CAD build for the part. Positions are in the model's coordinates, mm. Face numbers are marked on the shaded views. A direction names the side the tool comes from. Coordinates: 2 decimals unless noted, no trailing zeros. Order: outer loops, then holes, each group sorted by start corner. A loop starts at its lowest first (then second) coordinate and runs counter-clockwise, first axis right, second up. Notation, with made-up numbers: M 49,80.25 L 70,80.25 A24 cw 70,97.25 Z; hole C 36.25,-25.5 d3. An arc over 180 degrees is marked long. Write item = value, one per line.
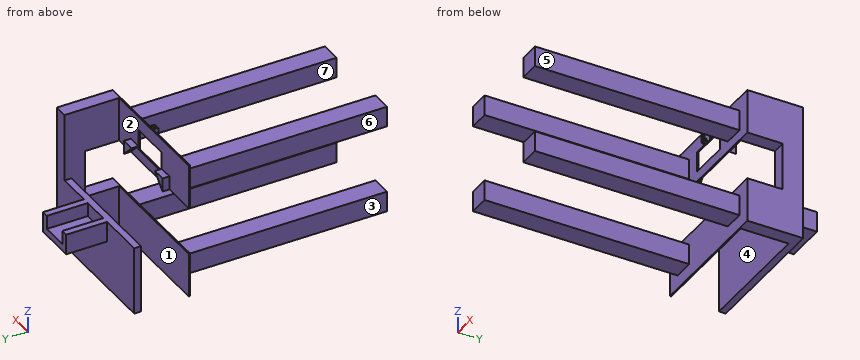
from build123d import *

# Parameters (mm, degrees)
SKETCH1_W           = 1000
SKETCH1_H           = 1000
BOSS_EXTRUDE1_DEPTH = 10
SKETCH5_W           = 150
SKETCH5_H           = 150
BOSS_EXTRUDE2_DEPTH = 1500
SKETCH7_W           = 300
SKETCH7_H           = 150
CUT_EXTRUDE1_DEPTH  = 1500
SKETCH9_W           = 10
SKETCH9_H           = 120
BOSS_EXTRUDE4_DEPTH = 40
FILLET1_R           = 10
FILLET2_R           = 10
SKETCH10_R          = 5
CUT_EXTRUDE3_DEPTH  = 55
SKETCH11_W          = 100
SKETCH11_H          = 1000
BOSS_EXTRUDE5_DEPTH = 400
SKETCH12_W          = 500
SKETCH12_H          = 50
BOSS_EXTRUDE6_DEPTH = 900
SKETCH14_W          = 300
SKETCH14_H          = 150
BOSS_EXTRUDE7_DEPTH = 300
SKETCH15_W          = 200
SKETCH15_H          = 100
CUT_EXTRUDE4_DEPTH  = 300
SKETCH8_W           = 1000
SKETCH8_H           = 350
CUT_EXTRUDE2_DEPTH  = 2069.840254829
SKETCH16_W          = 350
SKETCH16_H          = 250
CUT_EXTRUDE5_DEPTH  = 2062.552812809
BOSS_EXTRUDE8_DEPTH = 50
SKETCH21_R          = 7.5
CUT_EXTRUDE7_DEPTH  = 50
SKETCH22_R          = 7.5
CUT_EXTRUDE8_DEPTH  = 50


with BuildPart() as part:
    # Sketch1 → Boss-Extrude1 (new body)
    with BuildSketch(Plane(origin=(0, 0, 0), x_dir=(1, 0, 0), z_dir=(0, 1, 0))):
        with Locations((-500, 500)):
            Rectangle(SKETCH1_W, SKETCH1_H)
    extrude(amount=BOSS_EXTRUDE1_DEPTH)

    # Sketch5 → Boss-Extrude2 (add)
    with BuildSketch(Plane.XZ):
        with Locations((-825, -825)):
            Rectangle(SKETCH5_W, SKETCH5_H)
        with Locations((-825, -175)):
            Rectangle(SKETCH5_W, SKETCH5_H)
        with Locations((-175, -825)):
            Rectangle(SKETCH5_W, SKETCH5_H)
        with Locations((-175, -175)):
            Rectangle(SKETCH5_W, SKETCH5_H)
    extrude(amount=BOSS_EXTRUDE2_DEPTH)

    # Sketch7 → Cut-Extrude1 (cut)
    with BuildSketch(Plane(origin=(0, 10, 0), x_dir=(1, 0, 0), z_dir=(0, 1, 0))):
        with Locations((-500, 175)):
            Rectangle(SKETCH7_W, SKETCH7_H)
    extrude(amount=-CUT_EXTRUDE1_DEPTH, mode=Mode.SUBTRACT)

    # Sketch9 → Boss-Extrude4 (add)
    with BuildSketch(Plane.XZ):
        with Locations((-516, -60)):
            Rectangle(SKETCH9_W, SKETCH9_H)
        with Locations((-484, -60)):
            Rectangle(SKETCH9_W, SKETCH9_H)
    extrude(amount=BOSS_EXTRUDE4_DEPTH)

    # Fillet1
    fillet1_edges = [part.edges().sort_by_distance(p)[0] for p in [
        (-516, 0, -120),
        (-516, -40, -120),
        (-484, 0, -120),
        (-484, -40, -120),
    ]]
    fillet(fillet1_edges, radius=FILLET1_R)

    # Fillet2
    fillet2_edges = [part.edges().sort_by_distance(p)[0] for p in [
        (-516, -40, 0),
        (-484, -40, 0),
    ]]
    fillet(fillet2_edges, radius=FILLET2_R)

    # Sketch10 → Cut-Extrude3 (cut)
    with BuildSketch(Plane.ZY.offset(521)):
        with Locations((-110.273760932, -30.192862472)):
            Circle(SKETCH10_R)
    extrude(amount=-CUT_EXTRUDE3_DEPTH, mode=Mode.SUBTRACT)

    # Sketch11 → Boss-Extrude5 (add)
    with BuildSketch(Plane(origin=(0, 10, 0), x_dir=(1, 0, 0), z_dir=(0, 1, 0))):
        with Locations((-50, 500)):
            Rectangle(SKETCH11_W, SKETCH11_H)
    extrude(amount=BOSS_EXTRUDE5_DEPTH)

    # Sketch12 → Boss-Extrude6 (add)
    with BuildSketch(Plane.ZY.offset(100)):
        with Locations((-750, 385)):
            Rectangle(SKETCH12_W, SKETCH12_H)
    extrude(amount=BOSS_EXTRUDE6_DEPTH)

    # Sketch14 → Boss-Extrude7 (add)
    with BuildSketch(Plane(origin=(0, 410, 0), x_dir=(1, 0, 0), z_dir=(0, 1, 0))):
        with Locations((-500, 575)):
            Rectangle(SKETCH14_W, SKETCH14_H)
    extrude(amount=BOSS_EXTRUDE7_DEPTH)

    # Sketch15 → Cut-Extrude4 (cut)
    with BuildSketch(Plane(origin=(0, 710, 0), x_dir=(1, 0, 0), z_dir=(0, 1, 0))):
        with Locations((-500, 550)):
            Rectangle(SKETCH15_W, SKETCH15_H)
    extrude(amount=-CUT_EXTRUDE4_DEPTH, mode=Mode.SUBTRACT)

    # Sketch8 → Cut-Extrude2 (cut, through all)
    with BuildSketch(Plane(origin=(0, 10, 0), x_dir=(1, 0, 0), z_dir=(0, 1, 0))):
        with Locations((-500, 500)):
            Rectangle(SKETCH8_W, SKETCH8_H)
    extrude(amount=-CUT_EXTRUDE2_DEPTH, mode=Mode.SUBTRACT)

    # Sketch16 → Cut-Extrude5 (cut, through all)
    with BuildSketch(Plane(origin=(0, 0, 0), x_dir=(0, 0, -1), z_dir=(1, 0, 0))):
        with Locations((500, 135)):
            Rectangle(SKETCH16_W, SKETCH16_H)
    extrude(amount=-CUT_EXTRUDE5_DEPTH, mode=Mode.SUBTRACT)

    # Sketch18 → Boss-Extrude8 (add)
    with BuildSketch(Plane(origin=(0, 10, 0), x_dir=(1, 0, 0), z_dir=(0, 1, 0))):
        Polygon((-750, 325), (-750, 225), (-650, 225), align=None)
        Polygon((-350, 225), (-250, 225), (-250, 325), align=None)
    extrude(amount=BOSS_EXTRUDE8_DEPTH)

    # Sketch21 → Cut-Extrude7 (cut)
    with BuildSketch(Plane(origin=(-287.5, 0, -287.5), x_dir=(-0.7071067811865475, 0, 0.7071067811865477), z_dir=(-0.7071067811865477, 0, -0.7071067811865475))):
        with Locations((17.888347648, 45)):
            Circle(SKETCH21_R)
        with Locations((17.888347648, 25)):
            Circle(SKETCH21_R)
    extrude(amount=-CUT_EXTRUDE7_DEPTH, mode=Mode.SUBTRACT)

    # Sketch22 → Cut-Extrude8 (cut)
    with BuildSketch(Plane(origin=(-212.5, 0, 212.5), x_dir=(-0.7071067811865474, 0, -0.7071067811865477), z_dir=(0.7071067811865477, 0, -0.7071067811865474))):
        with Locations((689.218433538, 45)):
            Circle(SKETCH22_R)
        with Locations((689.218433538, 25)):
            Circle(SKETCH22_R)
    extrude(amount=-CUT_EXTRUDE8_DEPTH, mode=Mode.SUBTRACT)


solid = part.part
(1) Tool access for the marked faces 5, 6 and 7: list every direction of +Z, -Z, +X, -X, +Y, -Y with a clear straight run to the whole face (end or side of a thin tool).
Evaluation:
face_5 = +Z, -Z, +X, -Y
face_6 = +Z, -Z, -X, -Y
face_7 = +Z, -Z, -Y
(2) Pin check, flat tips, straight feed: pin 1 Ø24 at (x, z) = (-505.5, -74) entering from -Y; pin 2 Ø3 at (x, y) = (-486, -19) entering from -Z; pin 3 Ø20 at (y, z) = (-18, -44) entering from -X; pin 4 Ø11 at (x, y) = (-515.5, 2.5) entering from +Z. Stop position of each tip, or through.
Evaluation:
pin_1 = -40
pin_2 = -120
pin_3 = -521
pin_4 = 0
(3) Slice it at A-A, the plane x = -864.5. Write the cut outline in (y, z), then the cut area to 4 significant figures.
Evaluation:
outline = M -1500,-900 L 0,-900 L 0,-1000 L 10,-1000 L 10,-675 L 0,-675 L 0,-750 L -1500,-750 Z; M -1500,-250 L 0,-250 L 0,-325 L 10,-325 L 10,0 L 0,0 L 0,-100 L -1500,-100 Z; M 360,-1000 L 410,-1000 L 410,-500 L 360,-500 Z
area = 481,500 mm²
(4) Slice it at B-B, the plane y = -430. Write the cut outline in (x, z).
Evaluation:
outline = M -900,-900 L -750,-900 L -750,-750 L -900,-750 Z; M -900,-250 L -750,-250 L -750,-100 L -900,-100 Z; M -250,-900 L -100,-900 L -100,-750 L -250,-750 Z; M -250,-250 L -100,-250 L -100,-100 L -250,-100 Z
(5) Pull direction Y, two halves, no side cores. Call the marked faces 1, 2, 3 and 4: +Y half, -Y half, draft (parallel to the pull), parting line (faces both ways), or undercut.
Evaluation:
face_1 = undercut
face_2 = +Y half
face_3 = draft
face_4 = undercut
(6) Slice it at D-D, the plane x = -577. Write the cut outline in (y, z).
Evaluation:
outline = M 0,-1000 L 10,-1000 L 10,-675 L 0,-675 Z; M 0,-325 L 10,-325 L 10,-250 L 0,-250 Z; M 0,-100 L 10,-100 L 10,0 L 0,0 Z; M 360,-1000 L 410,-1000 L 410,-650 L 710,-650 L 710,-600 L 410,-600 L 410,-500 L 360,-500 Z
(7) Slice it at C-C, the plane z = -187.5. Write the cut outline in (x, y).
Evaluation:
outline = M -1000,0 L -900,0 L -900,-1500 L -750,-1500 L -750,0 L -650,0 L -650,10 L -1000,10 Z; M -350,0 L -250,0 L -250,-1500 L -100,-1500 L -100,0 L 0,0 L 0,410 L -100,410 L -100,10 L -350,10 Z
(8) Wall check: line 1 (X direction, y = 476.5, z = -506.5); line 2 (X direction, y = -740.5, z = -782.5). Give the ranges that are in metal, low to high. Write a range as from..to.
Evaluation:
line_1 = -650..-600, -400..-350
line_2 = -900..-750, -250..-100
